For this review, take the finished solid that the model builds, in its own axes (mm). A direction names the side the tool comes from. Give positions to 0.01 mm unless a question says otherwise; leave off trailing zeros. Order: outer loops, then holes, each group sorted by start corner. A loop starts at its lowest first (then second) coordinate and runs counter-clockwise, first axis right, second up. Notation, with made-up numbers: M 73,58.5 L 99,58.5 A11 ccw 99,75.5 Z; hole C -5,0 d1. An arc over 180 degrees is marked long. Answer as CSV lines item,"result". Start each with the question number.
1. Mouldability with a two-part tool opening along Z and no side actions: class faces 1 (the cylindrical face through (25.2, 24.61, 6.58)), 2 (the flat face through (24.15, 26, 4)), 3 (the flat face through (13, 17, 4)), 4 (the cylindrical face through (12.84, 6.41, -1.35)) as pulls with the +Z half, pulls with the -Z half, needs draft (parallel to the pull), parting line crosses it, or undercut.
2. We need section C-C, the plane y = 31.5. Give the boundary of the cut face in (x, z) (3 decimals), and give its area (3 significant figures).
3. For line 1 along X through (y, z) = (24, 5); line 2 along Z through (x, y) = (8.25, 19) (3 decimals); line 3 along Z through (x, y) = (12.9, 7.25), list the stretches that pass through material, from the lowest coordinate up.
4. We need section D-D, the plane z = 4. Give the boundary of the cut face in (x, y) (3 decimals), and give its area (3 significant figures).
5. Clearance check with flat-ended pins moving along their axes: P1, Ø6, axis at x = 5, y = 6.5, coming from the -Z side; P2, Ø14.5, axis at x = 14, y = 24.5, coming from the +Z side; P3, Ø2, axis at y = 27.5, z = 0.5, coming from the -X side; P4, Ø1.2, axis at x = 12.9, y = 24.75, coming from the -Z side. State where each tip first meets the part, or that it passes through.
6. Machinability: for faces 5 (the flat face through (13, 26, 1.925)), 6 (the flat face through (0, 25, 4)), 7 (the cylindrical face through (15.6, 6.66, 2.45)), which of the approach directions +Z, -Z, +X, -X, +Y, -Y give a long, thin tool a straight path to every point of the face, cutting with its end or side? Answer none if there is none.
7. We need section A-A, the plane y = 24.75. Give the boundary of the cut face in (x, z) (3 decimals), and give its area (3 significant figures).
8. We need section B-B, the plane x = 12.9. Give the boundary of the cut face in (y, z) (3 decimals), and give its area (3 significant figures).
from build123d import *

# Parameters (mm, degrees)
BOSS_EXTRUDE1_DEPTH = 7.15
SKETCH3_R           = 4.925
BOSS_EXTRUDE2_DEPTH = 15
SKETCH4_R           = 2.925
CUT_EXTRUDE1_DEPTH  = 13.5
SKETCH5_W           = 22.5
SKETCH5_H           = 3.3
CUT_EXTRUDE2_DEPTH  = 18
SKETCH6_R           = 1
CUT_EXTRUDE3_DEPTH  = 45.304514443
FILLET1_R           = 2


with BuildPart() as part:
    # Sketch2 → Boss-Extrude1 (new body)
    with BuildSketch(Plane.XY):
        Polygon((7.975, 0), (17.825, 0), (25.8, 14.5), (25.8, 35), (0, 35), (0, 14.5), align=None)
    extrude(amount=BOSS_EXTRUDE1_DEPTH)

    # Sketch3 → Boss-Extrude2 (add)
    with BuildSketch(Plane.XZ):
        with Locations((12.9, 3.575)):
            Circle(SKETCH3_R)
    extrude(amount=-BOSS_EXTRUDE2_DEPTH)

    # Sketch4 → Cut-Extrude1 (cut)
    with BuildSketch(Plane.XZ):
        with Locations((12.9, 3.575)):
            Circle(SKETCH4_R)
    extrude(amount=-CUT_EXTRUDE1_DEPTH, mode=Mode.SUBTRACT)

    # Sketch5 → Cut-Extrude2 (cut)
    with BuildSketch(Plane(origin=(0, 35, 0), x_dir=(1, 0, 0), z_dir=(0, 1, 0))):
        with Locations((12.9, -3.575)):
            Rectangle(SKETCH5_W, SKETCH5_H)
    extrude(amount=-CUT_EXTRUDE2_DEPTH, mode=Mode.SUBTRACT)

    # Sketch6 → Cut-Extrude3 (cut, through all)
    with BuildSketch(Plane(origin=(0, 0, 0), x_dir=(-1, 0, 0), z_dir=(0, 0, -1))):
        with Locations((-12.9, 24.75)):
            Circle(SKETCH6_R)
    extrude(amount=-CUT_EXTRUDE3_DEPTH, mode=Mode.SUBTRACT)

    # Fillet1
    # the kernel refuses this fillet: 2 mm, written as the material it takes off along each edge
    with BuildSketch(Plane(origin=(12.9, 15, 3.575), x_dir=(0.9794089200895291, 0, -0.20188652072157354), z_dir=(-0.20188652072157354, 0, -0.9794089200895291))) as fillet1_piece_1_section:
        with BuildLine():
            CenterArc((4.925 - FILLET1_R, FILLET1_R), FILLET1_R, 270, 90)
            Line((4.925 - FILLET1_R, 0), (4.925, 0))
            Line((4.925, 0), (4.925, FILLET1_R))
        make_face()
    fillet1_piece_1 = revolve(axis=Axis((12.9, 15, 3.575), (0, -1, 0)), revolution_arc=203.294598703, mode=Mode.PRIVATE)
    fillet1_piece_1 = split(fillet1_piece_1, bisect_by=Plane(origin=(12.9, 14.171762317, 7.15), z_dir=(0, 0, 1)), keep=Keep.TOP, mode=Mode.PRIVATE)
    add(fillet1_piece_1, mode=Mode.SUBTRACT)
    with BuildSketch(Plane(origin=(12.9, 15, 3.575), x_dir=(-0.9794089200895291, 0, 0.20188652072157326), z_dir=(0.20188652072157326, 0, 0.9794089200895291))) as fillet1_piece_2_section:
        with BuildLine():
            CenterArc((4.925 - FILLET1_R, FILLET1_R), FILLET1_R, 270, 90)
            Line((4.925 - FILLET1_R, 0), (4.925, 0))
            Line((4.925, 0), (4.925, FILLET1_R))
        make_face()
    fillet1_piece_2 = revolve(axis=Axis((12.9, 15, 3.575), (0, -1, 0)), revolution_arc=203.294598703, mode=Mode.PRIVATE)
    fillet1_piece_2 = split(fillet1_piece_2, bisect_by=Plane(origin=(12.9, 14.171762317, 0), z_dir=(0, 0, -1)), keep=Keep.TOP, mode=Mode.PRIVATE)
    add(fillet1_piece_2, mode=Mode.SUBTRACT)
    with BuildSketch(Plane(origin=(-2.409593749, 18.881079543, 7.15), x_dir=(0, 0, -1), z_dir=(0.48191874977215604, -0.876215908676647, 0))) as fillet1_piece_3_section:
        with BuildLine():
            CenterArc((FILLET1_R, FILLET1_R), FILLET1_R, 180, 90)
            Line((0, FILLET1_R), (0, 0))
            Line((0, 0), (FILLET1_R, 0))
        make_face()
    fillet1_piece_3 = extrude(amount=26.548432705, mode=Mode.PRIVATE)
    fillet1_piece_3 = fillet1_piece_3 - Plane(origin=(12.9, 7.738737356, 3.575), x_dir=(1, 0, 0), z_dir=(0, -1, 0)) * Cylinder(4.925, 62, mode=Mode.PRIVATE)
    add(fillet1_piece_3, mode=Mode.SUBTRACT)
    with BuildSketch(Plane(origin=(-2.409593749, 18.881079543, 0), x_dir=(0.876215908676647, 0.48191874977215604, 0), z_dir=(0.48191874977215604, -0.876215908676647, 0))) as fillet1_piece_4_section:
        with BuildLine():
            CenterArc((FILLET1_R, FILLET1_R), FILLET1_R, 180, 90)
            Line((0, FILLET1_R), (0, 0))
            Line((0, 0), (FILLET1_R, 0))
        make_face()
    fillet1_piece_4 = extrude(amount=26.548432705, mode=Mode.PRIVATE)
    fillet1_piece_4 = fillet1_piece_4 - Plane(origin=(12.9, 7.738737334, 3.575), x_dir=(1, 0, 0), z_dir=(0, -1, 0)) * Cylinder(4.925, 62, mode=Mode.PRIVATE)
    add(fillet1_piece_4, mode=Mode.SUBTRACT)
    with BuildSketch(Plane(origin=(15.415406251, -4.381079543, 7.15), x_dir=(-0.8762159086766471, 0.4819187497721556, 0), z_dir=(0.48191874977215565, 0.8762159086766471, 0))) as fillet1_piece_5_section:
        with BuildLine():
            CenterArc((FILLET1_R, -FILLET1_R), FILLET1_R, 90, 90)
            Line((0, -FILLET1_R), (0, 0))
            Line((0, 0), (FILLET1_R, 0))
        make_face()
    fillet1_piece_5 = extrude(amount=26.548432705, mode=Mode.PRIVATE)
    fillet1_piece_5 = fillet1_piece_5 - Plane(origin=(12.9, 7.738737334, 3.575), x_dir=(1, 0, 0), z_dir=(0, -1, 0)) * Cylinder(4.925, 62, mode=Mode.PRIVATE)
    add(fillet1_piece_5, mode=Mode.SUBTRACT)
    with BuildSketch(Plane(origin=(15.415406251, -4.381079543, 0), x_dir=(-0.8762159086766471, 0.4819187497721556, 0), z_dir=(0.48191874977215565, 0.8762159086766471, 0))) as fillet1_piece_6_section:
        with BuildLine():
            CenterArc((FILLET1_R, FILLET1_R), FILLET1_R, 180, 90)
            Line((0, FILLET1_R), (0, 0))
            Line((0, 0), (FILLET1_R, 0))
        make_face()
    fillet1_piece_6 = extrude(amount=26.548432705, mode=Mode.PRIVATE)
    fillet1_piece_6 = fillet1_piece_6 - Plane(origin=(12.9, 7.738737305, 3.575), x_dir=(1, 0, 0), z_dir=(0, -1, 0)) * Cylinder(4.925, 62, mode=Mode.PRIVATE)
    add(fillet1_piece_6, mode=Mode.SUBTRACT)
    with BuildSketch(Plane(origin=(25.8, 9.5, 7.15), x_dir=(-1, 0, 0), z_dir=(0, 1, 0)), Plane(origin=(0, 40, 7.15), x_dir=(1, 0, 0), z_dir=(0, -1, 0))) as fillet1_piece_7:
        with BuildLine():
            CenterArc((FILLET1_R, -FILLET1_R), FILLET1_R, 90, 90)
            Line((0, -FILLET1_R), (0, 0))
            Line((0, 0), (FILLET1_R, 0))
        make_face()
    extrude(amount=30.5, mode=Mode.SUBTRACT)
    with BuildSketch(Plane(origin=(0, 40, 0), x_dir=(1, 0, 0), z_dir=(0, -1, 0)), Plane(origin=(25.8, 9.5, 0), x_dir=(-1, 0, 0), z_dir=(0, 1, 0))) as fillet1_piece_8:
        with BuildLine():
            CenterArc((FILLET1_R, FILLET1_R), FILLET1_R, 180, 90)
            Line((0, FILLET1_R), (0, 0))
            Line((0, 0), (FILLET1_R, 0))
        make_face()
    extrude(amount=30.5, mode=Mode.SUBTRACT)


solid = part.part
Result set:
1,face 1,"pulls with the +Z half"
1,face 2,"undercut"
1,face 3,"undercut"
1,face 4,"pulls with the -Z half"
2,outline,"M 0,2 A2 ccw 2,0 L 23.8,0 A2 ccw 25.8,2 L 25.8,5.15 A2 ccw 23.8,7.15 L 2,7.15 A2 ccw 0,5.15 Z; hole M 1.65,1.925 L 24.15,1.925 L 24.15,5.225 L 1.65,5.225 Z"
2,area,"107 mm2"
3,line 1,"0 to 1.65, 24.15 to 25.8"
3,line 2,"0 to 1.925, 5.225 to 7.15"
3,line 3,"-1.35 to 0.65, 6.5 to 8.5"
4,outline,"M 0,14.5 L 7.975,0 L 10.006,0 L 10.006,13.5 L 15.794,13.5 L 15.794,0 L 17.825,0 L 25.8,14.5 L 25.8,35 L 24.15,35 L 24.15,17 L 1.65,17 L 1.65,35 L 0,35 Z"
4,area,"304 mm2"
5,P1,"z = 0"
5,P2,"z = 7.15"
5,P3,"x = 0.06"
5,P4,"through"
6,face 5,"+Y"
6,face 6,"+Z, -Z, -X, +Y, -Y"
6,face 7,"-Y"
7,outline,"M 0,2 A2 ccw 2,0 L 11.9,0 L 11.9,1.925 L 1.65,1.925 L 1.65,5.225 L 11.9,5.225 L 11.9,7.15 L 2,7.15 A2 ccw 0,5.15 Z; M 13.9,0 L 23.8,0 A2 ccw 25.8,2 L 25.8,5.15 A2 ccw 23.8,7.15 L 13.9,7.15 L 13.9,5.225 L 24.15,5.225 L 24.15,1.925 L 13.9,1.925 Z"
7,area,"99.1 mm2"
8,outline,"M 0,-1.35 L 13,-1.35 A2 ccw 14.891,0 L 23.75,0 L 23.75,1.925 L 17,1.925 L 17,5.225 L 23.75,5.225 L 23.75,7.15 L 14.891,7.15 A2 ccw 13,8.5 L 0,8.5 L 0,6.5 L 13.5,6.5 L 13.5,0.65 L 0,0.65 Z; M 25.75,0 L 35,0 L 35,1.925 L 25.75,1.925 Z; M 25.75,5.225 L 35,5.225 L 35,7.15 L 25.75,7.15 Z"
8,area,"143 mm2"
